Part model, mm, in its own coordinate system. Face numbers are marked on the shaded views. A direction names the side the tool comes from. Round coordinates to 2 decimals unless told otherwise and drop trailing zeros. Loops run counter-clockwise (first coordinate to the right, second up) from the corner with the lowest first, then second, coordinate; pieces in that order, holes last. Notation, with made-up numbers: M 43.5,69.5 L 48.5,69.5 A28 ccw 48.5,95.5 Z; hole C -15.5,40 d9. An arc over 180 degrees is marked long. Answer as CSV lines item,"result". Start each with the question number.
Item 1: Band-saw the part on C-C (y = 8.5). Give the cut face in (x, z), and give its area (3 significant figures).
Item 2: Drop flat-ended pins along their axis: pin 1 Ø10 at (x, y) = (23.5, 19.5) entering from +Z; pin 2 Ø4 at (x, y) = (13, 25.5) entering from +Z; pin 3 Ø4 at (x, y) = (18, 24.5) entering from -Z. Give the stop position or say it passes through.
Item 3: Band-saw the part on D-D (y = -7.5). Give the cut face in (x, z), and give its area (3 significant figures).
Item 4: Which spindle directions (+Z, -Z, +X, -X, +Y, -Y) get a long thin tool onto all of the face, cutting with end or side? Do the marked faces 4, 5 and 6. Say none if no direction does.
Item 5: Wall check: line 1 (Z direction, x = 0.85, y = 23.57); line 2 (Z direction, x = 1, y = 23); line 3 (X direction, y = 20, z = 26.5). Give the ranges that are in metal, low to high.
Item 6: Mould opens along Z. For the marked faces 1, 2 and 3 say: pulls with the +Z half, pulls with the -Z half, needs draft (parallel to the pull), parting line crosses it, or undercut.
Item 7: Band-saw the part on B-B (x = 28.5). Give the cut face in (y, z), and give its area (3 significant figures).
Item 8: Band-saw the part on A-A (z = 22.5). Give the cut face in (x, y).
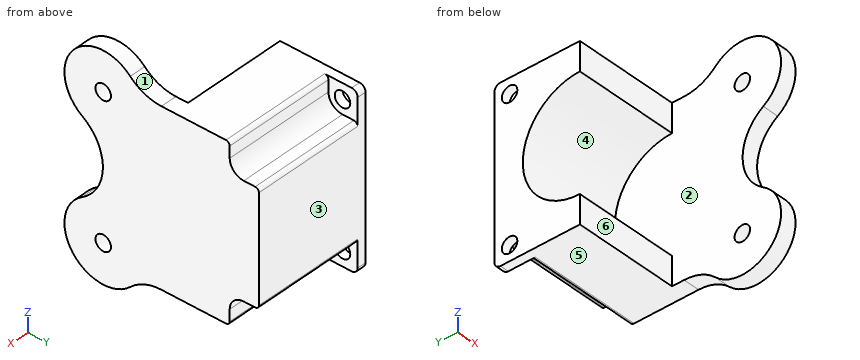
Autodesk Inventor part; units mm, degrees
ref_plane "YZ Plane" through (0, 0, 0) normal (1, 0, 0) x (0, 1, 0)
ref_plane "XZ Plane" through (0, 0, 0) normal (0, 1, 0) x (-1, 0, 0)
ref_plane "XY Plane" through (0, 0, 0) normal (0, 0, 1) x (1, 0, 0)
sketch "Sketch1" plane through (0, 0, 0) normal (1, 0, 0) x (0, 1, 0)
  arc A0 (0, -19.15) -> (0, 19.15) centre (0, 0) ccw
  line L0 (0, 28.65) -> (26.65, 28.65)
  line L1 (28.65, 26.65) -> (28.65, -26.65)
  line L2 (26.65, -28.65) -> (0, -28.65)
  line L3 (0, -28.65) -> (0, -19.15)
  line L4 (0, 19.15) -> (0, 28.65)
  arc A1 (28.65, 26.65) -> (26.65, 28.65) centre (26.65, 26.65) ccw
  arc A2 (26.65, -28.65) -> (28.65, -26.65) centre (26.65, -26.65) ccw
  line L5 (0, 23.57) -> (23.57, 23.57) construction
  line L6 (23.57, 23.57) -> (23.57, -23.57) construction
  line L7 (23.57, -23.57) -> (0, -23.57) construction
  line L8 (0, -23.57) -> (0, 23.57) construction
  circle A3 centre (23.57, 23.57) radius 2.6
  circle A4 centre (23.57, -23.57) radius 2.6
  point P0 (28.65, -28.65)
  point P1 (28.65, 28.65)
  dimension "d0" = 38.3
  dimension "d1" = 28.65
  dimension "d2" = 57.3
  dimension "d3" = 28.65
  dimension "d4" = 2
  dimension "d5" = 23.57
  dimension "d6" = 47.14
  dimension "d7" = 23.57
  dimension "d8" = 5.2
  dimension "d9" = 5.2
extrude "Extrusion1" add sketch "Sketch1" along normal blind 3
sketch "Sketch2" plane through (3, 0, 0) normal (1, 0, 0) x (0, 0, -1)
  circle A0 centre (-23.57, 23.57) radius 2.6
  circle A1 centre (23.57, 23.57) radius 2.6
  circle A2 centre (-23.57, 23.57) radius 4.72
  circle A3 centre (23.57, 23.57) radius 4.72
  line L0 (26.65, 28.65) -> (-26.65, 28.65)
  line L1 (-28.65, 26.65) -> (-28.65, 0)
  line L2 (28.65, 0) -> (28.65, 26.65)
  line L3 (26.65, 28.65) -> (-26.65, 28.65)
  arc A4 (-26.65, 28.65) -> (-28.65, 26.65) centre (-26.65, 26.65) ccw
  line L4 (-28.65, 26.65) -> (-28.65, 0)
  line L5 (-28.65, 0) -> (-19.15, 0)
  arc A5 (19.15, 0) -> (-19.15, 0) centre (0, 0) ccw
  line L6 (19.15, 0) -> (28.65, 0)
  line L7 (28.65, 0) -> (28.65, 26.65)
  arc A6 (28.65, 26.65) -> (26.65, 28.65) centre (26.65, 26.65) ccw
  circle A7 centre (-23.57, 23.57) radius 2.6
  circle A8 centre (23.57, 23.57) radius 2.6
  line L8 (-18.85, 28.65) -> (-18.85, 23.57)
  line L9 (-28.65, 18.85) -> (-23.57, 18.85)
  line L10 (18.85, 28.65) -> (18.85, 23.57)
  line L11 (28.65, 18.85) -> (23.57, 18.85)
  arc A9 (-17.6, 28.65) -> (-18.85, 27.4) centre (-17.6, 27.4) ccw
  arc A10 (-27.4, 18.85) -> (-28.65, 17.6) centre (-27.4, 17.6) ccw
  arc A11 (18.85, 27.4) -> (17.6, 28.65) centre (17.6, 27.4) ccw
  arc A12 (28.65, 17.6) -> (27.4, 18.85) centre (27.4, 17.6) ccw
  point P0 (-2.4769, -5.2226)
  point P1 (-57.3, 46.4)
  point P2 (-57.3, 10.9)
  point P3 (0, 10.9)
  point P4 (0, 46.4)
  point P5 (-10.9124, 57.3)
  point P6 (-46.3876, 57.3)
  dimension "d34" = 2.12
  dimension "d35" = 2.12
  dimension "d36" = 2.5
  dimension "d37" = 2.5
  dimension "d38" = 2.5
  dimension "d39" = 2.5
extrude "Extrusion2" add sketch "Sketch2" along normal blind 32 contours L8 A9 L0 A11 L10 A3 L11 A12 L2 L6 A5 L5 L1 A10 L9 A2
sketch "Sketch3" plane through (35, 0, 0) normal (1, 0, 0) x (0, 0, -1)
  circle A0 centre (-23.57, 23.57) radius 2.6 construction
  line L0 (-23.57, 23.57) -> (23.57, 23.57) construction
  line L1 (23.57, 23.57) -> (23.57, -23.57) construction
  line L2 (23.57, -23.57) -> (-23.57, -23.57) construction
  line L3 (-23.57, -23.57) -> (-23.57, 23.57) construction
  circle A1 centre (-23.57, -23.57) radius 2.6
  circle A2 centre (23.57, -23.57) radius 2.6
  arc A3 (-26.65, 28.65) -> (-28.65, 26.65) centre (-26.65, 26.65) ccw
  line L4 (-17.6, 28.65) -> (-26.65, 28.65)
  line L5 (17.6, 28.65) -> (-17.6, 28.65)
  line L6 (26.65, 28.65) -> (17.6, 28.65)
  arc A4 (28.65, 26.65) -> (26.65, 28.65) centre (26.65, 26.65) ccw
  line L7 (0, 0) -> (-7.096, 0) construction
  arc A5 (-28.65, -26.65) -> (-26.65, -28.65) centre (-26.65, -26.65) ccw
  line L8 (-20.0479, -28.65) -> (-26.65, -28.65)
  line L9 (26.65, -28.65) -> (20.0479, -28.65)
  arc A6 (26.65, -28.65) -> (28.65, -26.65) centre (26.65, -26.65) ccw
  line L10 (-28.65, 0) -> (-19.15, 0)
  line L11 (19.15, 0) -> (28.65, 0)
  line L12 (-28.65, 0) -> (-19.15, 0)
  line L13 (-28.65, 0) -> (-28.65, -26.65)
  line L14 (28.65, 0) -> (28.65, 17.6)
  line L15 (28.65, 0) -> (28.65, -26.65)
  arc A7 (16.0392, -27.1143) -> (-16.0392, -27.1143) centre (0, -44.9767) ccw
  arc A8 (-20.0479, -28.65) -> (-16.0392, -27.1143) centre (-20.0479, -22.65) ccw
  arc A9 (16.0392, -27.1143) -> (20.0479, -28.65) centre (20.0479, -22.65) ccw
  arc A10 (19.15, 0) -> (-19.15, 0) centre (0, 0) ccw
  line L16 (19.15, 0) -> (28.65, 0)
  line L17 (28.65, 0) -> (28.65, 17.6)
  arc A11 (28.65, 17.6) -> (27.4, 18.85) centre (27.4, 17.6) ccw
  line L18 (27.4, 18.85) -> (23.57, 18.85)
  arc A12 (18.85, 23.57) -> (23.57, 18.85) centre (23.57, 23.57) ccw
  line L19 (18.85, 23.57) -> (18.85, 27.4)
  arc A13 (18.85, 27.4) -> (17.6, 28.65) centre (17.6, 27.4) ccw
  line L20 (17.6, 28.65) -> (-17.6, 28.65)
  arc A14 (-17.6, 28.65) -> (-18.85, 27.4) centre (-17.6, 27.4) ccw
  line L21 (-18.85, 27.4) -> (-18.85, 23.57)
  arc A15 (-23.57, 18.85) -> (-18.85, 23.57) centre (-23.57, 23.57) ccw
  line L22 (-23.57, 18.85) -> (-27.4, 18.85)
  arc A16 (-27.4, 18.85) -> (-28.65, 17.6) centre (-27.4, 17.6) ccw
  line L23 (-28.65, 17.6) -> (-28.65, 0)
  line L24 (-28.65, 0) -> (-19.15, 0)
  circle A17 centre (23.57, -23.57) radius 13
  circle A18 centre (-23.57, -23.57) radius 13
  point P0 (-17.6, -28.65)
  point P1 (17.6, -28.65)
  point P2 (10.5708, -23.4226)
  point P3 (28.65, -11.6036)
  point P4 (-28.65, -11.6036)
  point P5 (-10.5708, -23.4226)
  dimension "d42" = 47.14
  dimension "d43" = 47.14
  dimension "d44" = 5.2
  dimension "d45" = 5.2
  dimension "d46" = 6
  dimension "d49" = 26
  dimension "d50" = 26
extrude "Extrusion3" add sketch "Sketch3" along normal blind 5.5
fillet "Fillet1" radius 15 4 edges at (37.75, -11.6036, 28.65) (37.75, -11.6036, -28.65) (37.75, -23.4226, 10.5708) (37.75, -23.4226, -10.5708)
equation "\"d9\" = d8"
equation "\"d37\" = d36"
equation "\"d38\" = d36"
equation "\"d39\" = d36"
properties part number "X Axis Pully Support"
Answer block:
1,outline,"M 0,-28.65 L 40.5,-28.65 L 40.5,28.65 L 0,28.65 L 0,17.16 L 35,17.16 L 35,-17.16 L 0,-17.16 Z"
1,area,"1,120 mm^2"
2,pin 1,"stops at z = 28.65"
2,pin 2,"stops at z = 18.85"
2,pin 3,"stops at z = -18.97"
3,outline,"M 35,-29.05 L 40.5,-29.05 L 40.5,29.05 L 35,29.05 Z"
3,area,"320 mm^2"
4,face 4,"-X, -Y"
4,face 5,"-Z, +X, -X, +Y"
4,face 6,"+Z, -Z, -X, -Y"
5,line 1,"z = -28.65 to -26.17, -20.97 to 20.97, 26.17 to 28.65"
5,line 2,"z = -28.65 to -26.11, -21.03 to 21.03, 26.11 to 28.65"
5,line 3,"x = 0 to 3"
6,face 1,"pulls with the +Z half"
6,face 2,"undercut"
6,face 3,"needs draft"
7,outline,"M 0,-28.65 L 17.6,-28.65 A1.25 ccw 18.85,-27.4 L 18.85,-23.57 A4.72 cw 23.57,-18.85 L 27.4,-18.85 A1.25 ccw 28.65,-17.6 L 28.65,17.6 A1.25 ccw 27.4,18.85 L 23.57,18.85 A4.72 cw 18.85,23.57 L 18.85,27.4 A1.25 ccw 17.6,28.65 L 0,28.65 L 0,19.15 A19.15 cw 0,-19.15 Z"
7,area,"882 mm^2"
8,outline,"M 0,0 L 35,0 L 35,-21.2 L 40.5,-21.2 L 40.5,18.97 L 3,18.97 L 3,21.2 L 0,21.2 Z; M 0,25.94 L 3,25.94 L 3,28.65 L 0,28.65 Z; M 35,-36.53 L 40.5,-36.53 L 40.5,-25.94 L 35,-25.94 Z"
